Verification items for the finished model (mm, model axes). A direction names the side the tool comes from. Give positions to 0.01 mm unless a question says otherwise; leave off trailing zeros. Order: outer loops, then holes, each group sorted by start corner. A loop starts at its lowest first (then second) coordinate and runs counter-clockwise, first axis right, second up. Notation, with made-up numbers: (4.5, -32.75) -> (28.5, -32.75) arc R24 ccw to (28.5, -2.75) -> close; hole circle Ø7 at (77.5, -33.75). An arc over 180 degrees is marked (long way). Write each question's results on one line, items separated by ' | '. Start each with the question number.
1. Depth check by flat-ended pin: pin 1 Ø10 at (x, y) = (-9, 376) entering from +Z; pin 2 Ø6 at (x, y) = (4.5, 647.5) entering from +Z; pin 3 Ø1 at (x, y) = (-15.5, 510) entering from -Z; pin 4 Ø12 at (x, z) = (-14.5, -11.5) entering from +Y. Enter the tip coordinate at first touch or a pass-through.
2. Set-up check for faces 1 (the face through (12.809, 493, -22.605)), 2 (the face through (24.981, 493, 0)): record each of +Z, -Z, +X, -X, +Y, -Y from which the full face is reachable in a straight line by a thin tool's end or side.
3. Mould release check, pull along X, two halves, no side actions. Record for faces 3 (the face through (25.981, 493, 0)), 4 (the face through (-12.316, 493, 21.735)), 5 (the face through (25.14, 1000, 0.14)): +X half, -X half, draft (parallel to the pull), parting line (faces both ways), or undercut.
4. Cross-section at A-A, the plane y = 548. Enter the section's corners in (x, z).
5. Cross-section at B-B, the plane z = 4.5. Enter the section's corners in (x, y), then the cut area to 3 significant figures.
6. Cross-section at C-C, the plane x = 17. Enter the section's corners in (y, z).
7. Material ranges on L1, parallel to Z at x = 0, y = 442; L2, parallel to X at y = 734.5, z = 13.5; L3, parallel to Z at x = -19.5, y = 438, recorded low to high. Write a range as from..to.
Solid Edge part; units mm, degrees
sketch "Sketch1" plane through (0, 0, 0) normal (0, -1, 0) x (1, 0, 0)
  line L0 (0, 30) -> (-25.9808, 15)
  line L1 (-25.9808, 15) -> (-25.9808, -15)
  line L2 (-25.9808, -15) -> (0, -30)
  line L3 (0, -30) -> (25.9808, -15)
  line L4 (25.9808, -15) -> (25.9808, 15)
  line L5 (25.9808, 15) -> (0, 30)
  line L6 (0, 28.8453) -> (-24.9808, 14.4226)
  line L7 (-24.9808, 14.4226) -> (-24.9808, -14.4226)
  line L8 (-24.9808, -14.4226) -> (0, -28.8453)
  line L9 (0, -28.8453) -> (24.9808, -14.4226)
  line L10 (24.9808, -14.4226) -> (24.9808, 14.4226)
  line L11 (24.9808, 14.4226) -> (0, 28.8453)
extrude "Protrusion1" add sketch "Sketch1" against normal blind 1000
Results below:
1) pin 1: stops at z = 27.69 | pin 2: stops at z = 29.13 | pin 3: stops at z = -21.34 | pin 4: passes through
2) face 1: -Z, +X, +Y, -Y | face 2: +Y, -Y
3) face 3: +X half | face 4: undercut | face 5: draft
4) outline: (-25.98, -15) -> (0, -30) -> (25.98, -15) -> (25.98, 15) -> (0, 30) -> (-25.98, 15) -> close; hole (-24.98, -14.42) -> (0, -28.85) -> (24.98, -14.42) -> (24.98, 14.42) -> (0, 28.85) -> (-24.98, 14.42) -> close
5) outline: (-25.98, 0) -> (-24.98, 0) -> (-24.98, 1000) -> (-25.98, 1000) -> close; (24.98, 0) -> (25.98, 0) -> (25.98, 1000) -> (24.98, 1000) -> close | area: 2,000 mm²
6) outline: (0, -20.19) -> (1000, -20.19) -> (1000, -19.03) -> (0, -19.03) -> close; (0, 19.03) -> (1000, 19.03) -> (1000, 20.19) -> (0, 20.19) -> close
7) L1: z = -30..-28.85, 28.85..30 | L2: x = -25.98..-24.98, 24.98..25.98 | L3: z = -18.74..-17.59, 17.59..18.74
